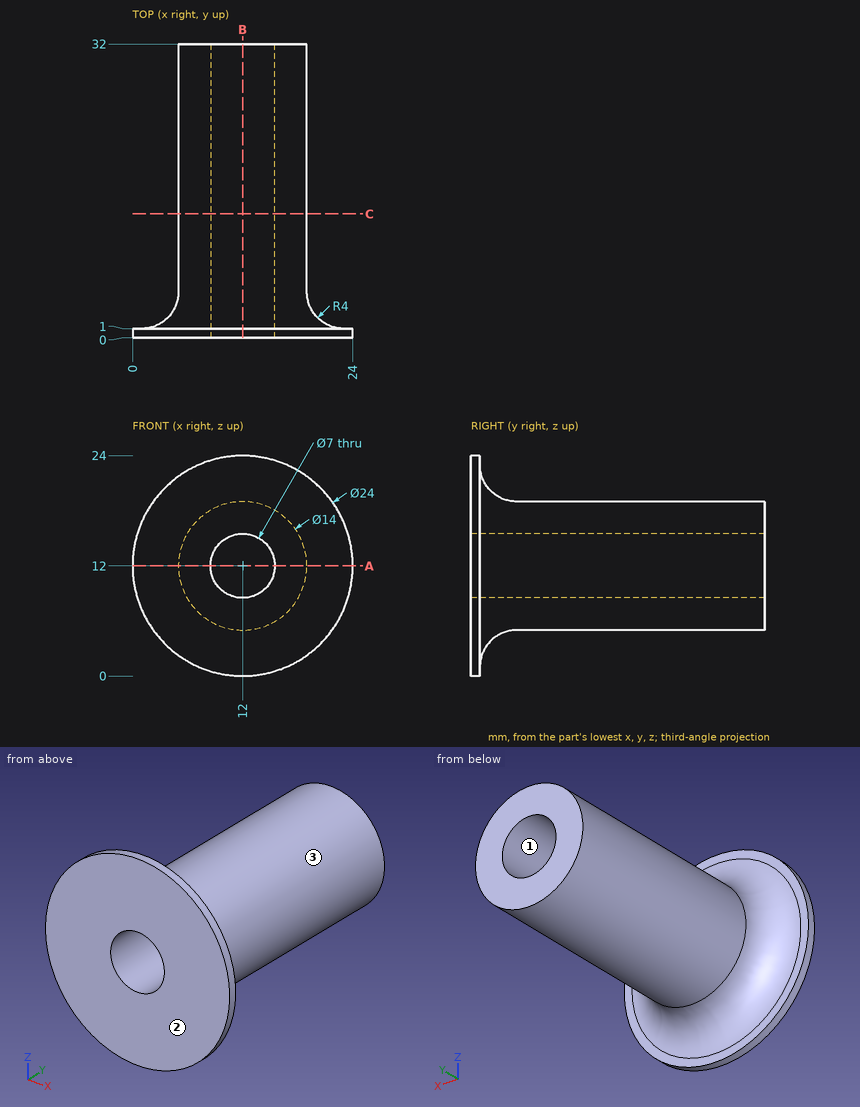
The figure shows three views and two pictorial views of one solid part (mm, origin at its lowest corner). Answer the questions. Give positions to 0.01 mm unless a question says otherwise; leave off trailing zeros. Write each loop counter-clockwise with the first axis right and the second up, starting at its lowest first coordinate (ties: lowest second). Pieces come first, ordered by that corner, then holes.
Q1. For a pull along Z with two mould halves and no side action, classify the marked faces 1, 2 and 3 as released by +Z, released by -Z, zero draft, split by the parting line, or undercut.
Answer:
face 1: undercut
face 2: zero draft
face 3: split by the parting line
Q2. Given pin 1 (4 mm diameter, centred on y = 23, z = 9, fed in from +X); pin 2 (1.5 mm diameter, centred on y = 6.5, z = 13.5, fed in from -X); pin 3 (1.5 mm diameter, centred on y = 25, z = 12, fed in from +X); pin 4 (6 mm diameter, centred on x = 16, z = 3.5, fed in from -Y), each flat-ended and moving along its own axis, determine where each tip first touches the part or whether it passes through.
Answer:
pin 1: stops at x = 18.93
pin 2: stops at x = 5.04
pin 3: stops at x = 19
pin 4: stops at y = 0
Q3. The part is cut by section C-C on y = 13.5. Give the vertices of the cut face in (x, z).
Answer:
outline: circle Ø14 at (12, 12); hole circle Ø7 at (12, 12)
Q4. The part is cut by section A-A on z = 12. Give the vertices of the cut face in (x, y), and give its area (3 significant figures).
Answer:
outline: (0, 0) - (8.5, 0) - (8.5, 32) - (5, 32) - (5, 5) arc R4 cw to (1, 1) - (0, 1) - close; (15.5, 0) - (24, 0) - (24, 1) - (23, 1) arc R4 cw to (19, 5) - (19, 32) - (15.5, 32) - close
area: 241 mm2
Q5. The part is cut by section B-B on x = 12. Give the vertices of the cut face in (y, z), and give its area (3 significant figures).
Answer:
outline: (0, 0) - (1, 0) - (1, 1) arc R4 cw to (5, 5) - (32, 5) - (32, 8.5) - (0, 8.5) - close; (0, 15.5) - (32, 15.5) - (32, 19) - (5, 19) arc R4 cw to (1, 23) - (1, 24) - (0, 24) - close
area: 241 mm2
Q6. Straight lines are drawn through the part: L1, parallel to X at y = 13, z = 12; L2, parallel to Z at x = 12.75, y = 21.5. For each, find the intervals that lie inside material, in ascending order.
Answer:
L1: x = 5 to 8.5, 15.5 to 19
L2: z = 5.04 to 8.58, 15.42 to 18.96
